Input: part model. Units: mm. Frame: model coordinates. Coordinates: 2 decimals unless noted, no trailing zeros. Loops run counter-clockwise (first coordinate to the right, second up) from the corner with the lowest first, then second, coordinate; pieces in that order, holes last.
```python
from build123d import *

# Parameters (mm, degrees)
SKETCH1_W           = 762
SKETCH1_H           = 762
BOSS_EXTRUDE1_DEPTH = 2.38125
CUT_EXTRUDE1_DEPTH  = 3.38125


with BuildPart() as part:
    # Sketch1 → Boss-Extrude1 (new body)
    with BuildSketch(Plane(origin=(0, 0, 0), x_dir=(1, 0, 0), z_dir=(0, 1, 0))):
        Rectangle(SKETCH1_W, SKETCH1_H)
    extrude(amount=BOSS_EXTRUDE1_DEPTH)

    # Sketch2 → Cut-Extrude1 (cut, through all)
    with BuildSketch(Plane(origin=(0, 2.38125, 0), x_dir=(1, 0, 0), z_dir=(0, 1, 0))):
        with BuildLine():
            Line((234.95, 381), (381, 381))
            Line((381, 381), (381, 234.95))
            ThreePointArc((381, 234.95), (277.727054608, 277.727054608), (234.95, 381))
        make_face()
        with BuildLine():
            Line((381, -234.95), (381, -381))
            Line((381, -381), (234.95, -381))
            ThreePointArc((234.95, -381), (277.727054608, -277.727054608), (381, -234.95))
        make_face()
        with BuildLine():
            Line((-234.95, -381), (-381, -381))
            Line((-381, -381), (-381, -234.95))
            ThreePointArc((-381, -234.95), (-277.727054608, -277.727054608), (-234.95, -381))
        make_face()
        with BuildLine():
            Line((-381, 234.95), (-381, 381))
            Line((-381, 381), (-234.95, 381))
            ThreePointArc((-234.95, 381), (-277.727054608, 277.727054608), (-381, 234.95))
        make_face()
    extrude(amount=-CUT_EXTRUDE1_DEPTH, mode=Mode.SUBTRACT)


solid = part.part
```
Item 1: Line query: L1, parallel to X at y = 1.35, z = 325; L2, parallel to Z at x = 254.5, y = 1.5; L3, parallel to X at y = 1.3, z = -276.5. Output: solid intervals per line, ascending.
Result:
L1: x = -246.11 to 246.11
L2: z = -308 to 308
L3: x = -278.97 to 278.97
Item 2: Section query A-A (y = 1.35). Output: boundary loops of the cut face in (x, z), then the cut area to 3 significant figures.
Result:
outline: (-381, -234.95) arc R146.05 cw to (-234.95, -381) - (234.95, -381) arc R146.05 cw to (381, -234.95) - (381, 234.95) arc R146.05 cw to (234.95, 381) - (-234.95, 381) arc R146.05 cw to (-381, 234.95) - close
area: 514,000 mm2
Item 3: Section query B-B (z = 325.5). Output: boundary loops of the cut face in (x, y), then the cut area to 3 significant figures.
Result:
outline: (-245.91, 0) - (245.91, 0) - (245.91, 2.38) - (-245.91, 2.38) - close
area: 1,170 mm2
Item 4: Section query C-C (x = 288). Output: boundary loops of the cut face in (y, z).
Result:
outline: (0, -268.39) - (2.38, -268.39) - (2.38, 268.39) - (0, 268.39) - close
